```python
from build123d import *


with BuildPart() as part:
    # Sketch1 → Revolve1 (revolve)
    with BuildSketch(Plane(origin=(0, 0, 0), x_dir=(0, 0, -1), z_dir=(1, 0, 0)), mode=Mode.PRIVATE) as revolve1_sk:
        Polygon((2.9718, 10.95375), (-2.9718, 10.95375), (-2.9718, 9.3091), (-5.4356, 9.3091), (-5.4356, 8.128), (-2.2606, 8.128), (-2.2606, 4.4958), (-5.4356, 4.4958), (-5.4356, 3.3147), (1.1938, 3.3147), (1.1938, 1.55575), (13.8684, 1.55575), (13.8684, 3.2512), (2.2225, 3.2512), (2.2225, 4.4958), (-0.5207, 4.4958), (-0.5207, 8.128), (5.4356, 8.128), (5.4356, 9.3091), (2.9718, 9.3091), align=None)
    revolve(revolve1_sk.sketch.rotate(Axis((0, 0, 0), (0, 0, 1)), 90), axis=Axis((0, 0, 0), (0, 0, 1)))


solid = part.part
```
Design review of the part built by this model. Coordinates are the model's own, in mm. A direction names the side the tool comes from. Give positions to 0.01 mm unless a question says otherwise; leave off trailing zeros. Order: outer loops, then holes, each group sorted by start corner. A loop starts at its lowest first (then second) coordinate and runs counter-clockwise, first axis right, second up. Notation, with made-up numbers: (81.25, 83.5) - (121.25, 83.5) arc R18 cw to (121.25, 109.5) - close; hole circle Ø2 at (35.5, -6.75). An arc over 180 degrees is marked (long way). Use a Markdown table: item, result. Add a question column.
(1) Add section A-A on y = 3.75. Give the boundary of the cut face in (x, z), then the cut area to 3 significant figures.
(2) Add section C-C on z = -11.25. Give the boundary of the cut face in (x, y), then the cut area to 3 significant figures.
(3) Add section D-D on y = -4. Give the boundary of the cut face in (x, z).
(4) Clearance check with flat-ended pins moving along their axes: P1, Ø4, axis at x = 0, y = 0, coming from the +Z side; P2, Ø3, axis at y = 4.5, z = -12, coming from the -X side; P3, Ø2, axis at x = 7, y = 8, coming from the +Z side. State where each tip first meets the part, or that it passes through.
(5) Machinability: for faces 5 (the face through (-8.88, -2.8, -4.19)), 6 (the face through (4.9, 8.1, 2.972)), 7 (the face through (-0.72, 1.38, -7.62)), which of the approach directions +Z, -Z, +X, -X, +Y, -Y give a long, thin tool a straight path to every point of the face, cutting with its end or side? Answer none if there is none.
(6) Wall thickness on probe 1 along Y at (x, z) = (0, -4); probe 2 along Y at (x, z) = (0, 3.85); probe 3 along Z at (x, y) = (-5.5, 6.5): over which ranges is each line inside the solid? List them lowest first. Write a range as [from, to].
(7) Add section B-B on x = 6.5. Give the boundary of the cut face in (y, z), then the cut area to 3 significant figures.
(8) Mouldability with a two-part tool opening along Y and no side actions: class faces 1 (the face through (2.375, 10.693, 0.042)), 2 (the face through (0.97, 4.39, -0.83)), 3 (the face through (1.762, 7.935, 3.826)), 4 (the face through (2, 3, 5.436)) as +Y half, -Y half, draft (parallel to the pull), parting line (faces both ways), or undercut.
Report:
| question | item | result |
|---|---|---|
| 1 | outline | (-10.29, -2.97) - (-8.52, -2.97) - (-8.52, -5.44) - (-7.21, -5.44) - (-7.21, 0.52) - (-2.48, 0.52) - (-2.48, -2.22) - (2.48, -2.22) - (2.48, 0.52) - (7.21, 0.52) - (7.21, -5.44) - (8.52, -5.44) - (8.52, -2.97) - (10.29, -2.97) - (10.29, 2.97) - (8.52, 2.97) - (8.52, 5.44) - (7.21, 5.44) - (7.21, 2.26) - (2.48, 2.26) - (2.48, 5.44) - (-2.48, 5.44) - (-2.48, 2.26) - (-7.21, 2.26) - (-7.21, 5.44) - (-8.52, 5.44) - (-8.52, 2.97) - (-10.29, 2.97) - close |
| 1 | area | 104 mm² |
| 2 | outline | circle Ø6.5 at (0, 0); hole circle Ø3.11 at (0, 0) |
| 2 | area | 25.6 mm² |
| 3 | outline | (-10.2, -2.97) - (-8.41, -2.97) - (-8.41, -5.44) - (-7.08, -5.44) - (-7.08, 0.52) - (-2.05, 0.52) - (-2.05, -2.22) - (2.05, -2.22) - (2.05, 0.52) - (7.08, 0.52) - (7.08, -5.44) - (8.41, -5.44) - (8.41, -2.97) - (10.2, -2.97) - (10.2, 2.97) - (8.41, 2.97) - (8.41, 5.44) - (7.08, 5.44) - (7.08, 2.26) - (2.05, 2.26) - (2.05, 5.44) - (-2.05, 5.44) - (-2.05, 2.26) - (-7.08, 2.26) - (-7.08, 5.44) - (-8.41, 5.44) - (-8.41, 2.97) - (-10.2, 2.97) - close |
| 4 | P1 | stops at z = -1.19 |
| 4 | P2 | stops at x = -1.25 |
| 4 | P3 | stops at z = 2.97 |
| 5 | face 5 | -Z |
| 5 | face 6 | +Z |
| 5 | face 7 | +Z, -Z |
| 6 | probe 1 | y = [-9.31, -8.13], [-3.25, -1.56], [1.56, 3.25], [8.13, 9.31] |
| 6 | probe 2 | y = [-9.31, -8.13], [-4.5, -3.31], [3.31, 4.5], [8.13, 9.31] |
| 6 | probe 3 | z = [-5.44, 5.44] |
| 7 | outline | (-8.82, -2.97) - (-6.66, -2.97) - (-6.66, -5.44) - (-4.88, -5.44) - (-4.88, 0.52) - (4.88, 0.52) - (4.88, -5.44) - (6.66, -5.44) - (6.66, -2.97) - (8.82, -2.97) - (8.82, 2.97) - (6.66, 2.97) - (6.66, 5.44) - (4.88, 5.44) - (4.88, 2.26) - (-4.88, 2.26) - (-4.88, 5.44) - (-6.66, 5.44) - (-6.66, 2.97) - (-8.82, 2.97) - close |
| 7 | area | 81.4 mm² |
| 8 | face 1 | parting line |
| 8 | face 2 | undercut |
| 8 | face 3 | undercut |
| 8 | face 4 | draft |
